Autodesk Inventor part; units mm, degrees
ref_plane "YZ Plane" through (0, 0, 0) normal (1, 0, 0) x (0, 1, 0)
ref_plane "XZ Plane" through (0, 0, 0) normal (0, 1, 0) x (-1, 0, 0)
ref_plane "XY Plane" through (0, 0, 0) normal (0, 0, 1) x (1, 0, 0)
ref_plane "Work Plane1" through (1.0737, -2.7207, -1.3848) normal (0, 0, 1) x (1, 0.0049, 0)
sketch "Sketch1" plane through (1.0737, -2.7207, -1.3848) normal (0, 0, 1) x (1, 0.0049, 0)
  line L0 (-12.5, -4.85) -> (-12.5, 4.35)
  line L1 (12.5, 4.35) -> (12.5, -4.85)
  line L2 (11.5, -5.85) -> (-11.5, -5.85)
  circle A0 centre (8.5, 0.85) radius 3
  circle A1 centre (-8.5, 0.85) radius 3
  circle A2 centre (0, -2.15) radius 1.1
  line L3 (4.0694, -5.85) -> (-4.0694, -5.85)
  circle A3 centre (0, -2.15) radius 1.1
  line L4 (-11.5, 5.35) -> (11.5, 5.35)
  arc A4 (-12.5, -4.85) -> (-11.5, -5.85) centre (-11.5, -4.85) ccw
  arc A5 (-11.5, 5.35) -> (-12.5, 4.35) centre (-11.5, 4.35) ccw
  arc A6 (12.5, 4.35) -> (11.5, 5.35) centre (11.5, 4.35) ccw
  arc A7 (11.5, -5.85) -> (12.5, -4.85) centre (11.5, -4.85) ccw
  point P0 (-1.0602, 2.726)
  dimension "d0" = 2.2
extrude "Extrusion1" add sketch "Sketch1" along normal mid plane 4
sketch "Sketch2" plane through (1.0737, -2.7207, 0.6152) normal (0, 0, 1) x (1, 0.0049, 0)
  line L0 (-12.5, 4.35) -> (-12.5, -4.85)
  line L1 (-11.5, -5.85) -> (11.5, -5.85)
  line L2 (12.5, -4.85) -> (12.5, 4.35)
  circle A0 centre (8.5, 0.85) radius 3
  circle A1 centre (-8.5, 0.85) radius 3
  line L3 (11.5, 0.85) -> (12.5, 0.85)
  line L4 (12.5, -4.85) -> (12.5, 4.35)
  circle A2 centre (8.5, 0.85) radius 3
  line L5 (8.5, 3.85) -> (0.045, 5.85)
  line L6 (12.5, 5.85) -> (-12.5, 5.85)
  circle A3 centre (0, -2.15) radius 1.1
  line L7 (11.5, 5.35) -> (-11.5, 5.35)
  arc A4 (-12.5, -4.85) -> (-11.5, -5.85) centre (-11.5, -4.85) ccw
  arc A5 (11.5, -5.85) -> (12.5, -4.85) centre (11.5, -4.85) ccw
  arc A6 (12.5, 4.35) -> (11.5, 5.35) centre (11.5, 4.35) ccw
  arc A7 (-11.5, 5.35) -> (-12.5, 4.35) centre (-11.5, 4.35) ccw
  point P0 (-1.0602, 2.726)
  point P1 (-12.5, 5.85)
  point P2 (8.5, 3.85)
  point P3 (12.5, 0.85)
extrude "Extrusion2" [suppressed]
sketch "Sketch3" plane through (1.0737, -2.7207, 0.6152) normal (0, 0, 1) x (1, 0.0049, 0)
  line L0 (-12.5, 4.35) -> (-12.5, -4.85)
  line L1 (-11.5, -5.85) -> (11.5, -5.85)
  line L2 (12.5, -4.85) -> (12.5, 4.35)
  circle A0 centre (8.5, 0.85) radius 3
  circle A1 centre (-8.5, 0.85) radius 3
  circle A2 centre (0, -2.15) radius 1.1
  line L3 (-12.5, 4.35) -> (-12.5, -4.85)
  line L4 (-12.5, 5.85) -> (-9.6209, 5.85)
  line L5 (-9.6209, 5.85) -> (-9.6209, 5.35)
  line L6 (-9.6209, 5.35) -> (-12.5, 5.35)
  line L7 (-12.5, 5.35) -> (-12.5, 5.85)
  line L8 (-12.5, 5.85) -> (7.0362, 5.85)
  line L9 (7.0362, 5.85) -> (7.0362, 5.35)
  line L10 (7.0362, 5.35) -> (-12.5, 5.35)
  line L11 (-12.5, 5.35) -> (-12.5, 5.85)
  arc A3 (12.5, 4.35) -> (11.5, 5.35) centre (11.5, 4.35) ccw
  line L12 (11.5, 5.35) -> (-11.5, 5.35)
  arc A4 (-11.5, 5.35) -> (-12.5, 4.35) centre (-11.5, 4.35) ccw
  arc A5 (-12.5, -4.85) -> (-11.5, -5.85) centre (-11.5, -4.85) ccw
  arc A6 (11.5, -5.85) -> (12.5, -4.85) centre (11.5, -4.85) ccw
  point P0 (-1.0602, 2.726)
  point P1 (-12.5, -5.85)
  point P2 (-12.5, 5.35)
  point P3 (-9.6209, 5.35)
  point P4 (-11.5, 5.35)
  point P5 (-12.5, 5.35)
  point P6 (-9.6209, 5.35)
  point P7 (7.0362, 5.35)
  point P8 (7.0362, 5.35)
  dimension "d5" = 0.5
extrude "Extrusion3" cut sketch "Sketch3" against normal blind 10 contours A4 L6 L10 L12 A3 L2 A6 L1 A5 L0 | L6 L7 L4 L5 | L5 L8 L9 L10 | A1 | A2
sketch "Sketch4" plane through (1.0737, -2.7207, -1.3848) normal (0, 0, 1) x (1, 0.0049, 0)
  arc A0 (-12.5, -4.85) -> (-11.5, -5.85) centre (-11.5, -4.85) ccw
  line L0 (-11.5, -5.85) -> (11.5, -5.85)
  arc A1 (11.5, -5.85) -> (12.5, -4.85) centre (11.5, -4.85) ccw
  line L1 (12.5, -4.85) -> (12.5, 4.35)
  arc A2 (12.5, 4.35) -> (11.5, 5.35) centre (11.5, 4.35) ccw
  line L2 (11.5, 5.35) -> (-11.5, 5.35)
  arc A3 (-11.5, 5.35) -> (-12.5, 4.35) centre (-11.5, 4.35) ccw
  line L3 (-12.5, 4.35) -> (-12.5, -4.85)
  circle A4 centre (0, -2.15) radius 1.1
  circle A5 centre (8.5, 0.85) radius 3
  circle A6 centre (-8.5, 0.85) radius 3
  line L4 (8.5, 3.85) -> (4.0971, 5.35)
  line L5 (11.5, 0.85) -> (12.5, -4.85)
  point P0 (-1.0602, 2.726)
extrude "Extrusion4" add sketch "Sketch4" along normal mid plane 3 contours L3 A3 L2 L4 A5 L5 A1 L0 A0
properties part number "srodek"
Could you check a few things on this model? Use its own coordinates, in mm. Give positions to 0.01 mm unless a question says otherwise; leave off trailing zeros. Order: outer loops, then holes, each group sorted by start corner. A loop starts at its lowest first (then second) coordinate and runs counter-clockwise, first axis right, second up.
Q1. Suppose I cut it at B-B, the plane x = 1. Write out the boundary of the cut face in (y, z), and give its area (3 significant figures).
Q2. Suppose I cut it at D-D, the plane y = -4.5. Write out the boundary of the cut face in (x, z), and give its area (3 significant figures).
Q3. I'm going to push flat-ended pins straight in: P1, Ø1, axis at y = -4, z = -2.5, coming from the +X side; P2, Ø1.5, axis at x = 2, z = -2.5, coming from the +Y side. Where does each tip first touch, or does it pass through?
Q4. If I drill on line 1 along X through (y, z) = (-3.5, -1); line 2 along X through (y, z) = (-2.75, -2.5); line 3 along X through (y, z) = (-4, -2), over which ranges is the centre line in solid material (lowest first)?
Q5. Suppose I cut it at A-A, the plane y = -1. Write out the boundary of the cut face in (x, z).
Q6. Suppose I cut it at C-C, the plane z = -1.75. Write out the boundary of the cut face in (x, y), and give its area (3 significant figures).
Q7. We'd pull the mould along X, two halves only. Please class faces 1 (the cylindrical face through (13.316, -8.21, -1.406)), 2 (the flat face through (1, -3, 0.115)), 3 (the cylindrical face through (-10.427, -2.059, -1.406)): +X half, -X half, draft (parallel to the pull), parting line (faces both ways), or undercut.
Solution:
1. outline: (-8.57, -2.88) - (-5.97, -2.88) - (-5.97, 0.12) - (-8.57, 0.12) - close; (-3.77, -2.88) - (2.63, -2.88) - (2.63, 0.12) - (-3.77, 0.12) - close
1. area: 27.0 mm2
2. outline: (-11.42, -2.88) - (-8.95, -2.88) - (-8.95, 0.12) - (-11.42, 0.12) - close; (-5.91, -2.88) - (0.05, -2.88) - (0.05, 0.12) - (-5.91, 0.12) - close; (2.12, -2.88) - (8.2, -2.88) - (8.2, 0.12) - (2.12, 0.12) - close; (10.94, -2.88) - (13.05, -2.88) - (13.05, 0.12) - (10.94, 0.12) - close
2. area: 49.9 mm2
3. P1: stops at x = 13.05
3. P2: stops at y = 2.64
4. line 1: x = -11.42 to -9.98, -4.88 to 7.08, 12.06 to 12.87
4. line 2: x = -11.43 to -10.31, -4.55 to 6.71, 12.42 to 12.74
4. line 3: x = -11.42 to -9.58, -5.28 to 0.41, 1.76 to 7.5, 11.64 to 12.96
5. outline: (-11.43, -2.88) - (-10.29, -2.88) - (-10.29, 0.12) - (-11.43, 0.12) - close; (-4.57, -2.88) - (6.69, -2.88) - (6.69, 0.12) - (-4.57, 0.12) - close
6. outline: (-11.45, 1.57) - (-11.4, -7.63) arc R1 ccw to (-10.4, -8.63) - (12.6, -8.51) arc R1 ccw to (13.6, -7.51) - (12.57, -1.81) arc R3 cw (long way) to (9.55, 1.17) - (5.14, 2.65) - (-10.45, 2.57) arc R1 ccw to start; hole circle Ø6 at (-7.43, -1.91); hole circle Ø2.2 at (1.08, -4.87)
6. area: 202 mm2
7. face 1: +X half
7. face 2: draft
7. face 3: undercut
